Check sheet for the modelled part. Datum: model origin and axes. Units: mm. A direction names the side the tool comes from. Coordinates: 2 decimals unless noted, no trailing zeros. Order: outer loops, then holes, each group sorted by start corner. A loop starts at its lowest first (then second) coordinate and runs counter-clockwise, first axis right, second up.
from build123d import *

# Parameters (mm, degrees)
SKETCH_1_W      = 11.5
SKETCH_1_H      = 30
SKETCH_1_W_2    = 3
SKETCH_1_W_3    = 18.5
SKETCH_1_W_4    = 200
EXTRUDE_3_DEPTH = 5
FILLET_2_R      = 2


with BuildPart() as part:
    # 草图1 → 凸台-拉伸3 (new body)
    # profile 1 of 4: a face of its own
    with BuildSketch(Plane(origin=(0, 0, 0), x_dir=(0, 0, -1), z_dir=(1, 0, 0))):
        Rectangle(SKETCH_1_W, SKETCH_1_H)
        with BuildLine():
            Line((-1.75, -10), (-1.75, 10))
            ThreePointArc((-1.75, 10), (0, 11.75), (1.75, 10))
            Line((1.75, 10), (1.75, -10))
            ThreePointArc((1.75, -10), (0, -11.75), (-1.75, -10))
        make_face(mode=Mode.SUBTRACT)
    # profile 2 of 4: a face of its own
    with BuildSketch(Plane(origin=(0, 0, 0), x_dir=(0, 0, -1), z_dir=(1, 0, 0))):
        with Locations((-7.25, 0)):
            Rectangle(SKETCH_1_W_2, SKETCH_1_H)
    # profile 3 of 4: a face of its own
    with BuildSketch(Plane(origin=(0, 0, 0), x_dir=(0, 0, -1), z_dir=(1, 0, 0))):
        with Locations((15, 0)):
            Rectangle(SKETCH_1_W_3, SKETCH_1_H)
        with BuildLine():
            ThreePointArc((20.25, -10), (18.5, -11.75), (16.75, -10))
            Line((16.75, -10), (16.75, 10))
            ThreePointArc((16.75, 10), (18.5, 11.75), (20.25, 10))
            Line((20.25, 10), (20.25, -10))
        make_face(mode=Mode.SUBTRACT)
    # profile 4 of 4: a face of its own
    with BuildSketch(Plane(origin=(0, 0, 0), x_dir=(0, 0, -1), z_dir=(1, 0, 0))):
        with Locations((124.25, 0)):
            Rectangle(SKETCH_1_W_4, SKETCH_1_H)
        with BuildLine():
            ThreePointArc((36, -10), (34.25, -11.75), (32.5, -10))
            Line((32.5, -10), (32.5, 10))
            ThreePointArc((32.5, 10), (34.25, 11.75), (36, 10))
            Line((36, 10), (36, -10))
        make_face(mode=Mode.SUBTRACT)
        with BuildLine():
            ThreePointArc((51, -10), (49.25, -11.75), (47.5, -10))
            Line((47.5, -10), (47.5, 10))
            ThreePointArc((47.5, 10), (49.25, 11.75), (51, 10))
            Line((51, 10), (51, -10))
        make_face(mode=Mode.SUBTRACT)
        with BuildLine():
            ThreePointArc((196, -10), (194.25, -11.75), (192.5, -10))
            Line((192.5, -10), (192.5, 10))
            ThreePointArc((192.5, 10), (194.25, 11.75), (196, 10))
            Line((196, 10), (196, -10))
        make_face(mode=Mode.SUBTRACT)
        with BuildLine():
            ThreePointArc((207.5, 10), (209.25, 11.75), (211, 10))
            Line((211, 10), (211, -10))
            ThreePointArc((211, -10), (209.25, -11.75), (207.5, -10))
            Line((207.5, -10), (207.5, 10))
        make_face(mode=Mode.SUBTRACT)
    extrude(amount=EXTRUDE_3_DEPTH)

    # 圆角2
    fillet_2_edges = [part.edges().sort_by_distance(p)[0] for p in [
        (0, 0, 8.75),
    ]]
    fillet(fillet_2_edges, radius=FILLET_2_R)


solid = part.part
(1) Tool access check on faces 1 (the flat face through (0, 0, -107)), 2 (the flat face through (2, 0, -196)). Record the directions out of +Z, -Z, +X, -X, +Y, -Y that give a thin tool (end or side, any length) a straight path to the whole face; none if there is none.
Filled in:
face 1: +Z, -Z, -X, +Y, -Y
face 2: +X, -X
(2) Release check for a two-part mould opening along Y. For faces 3 (the flat face through (2, 0, -32.5)), 4 (the flat face through (2, 0, -224.25)), 5 (the flat face through (2, -15, -106)) record: +Y half, -Y half, draft (parallel to the pull), parting line (faces both ways), or undercut.
Filled in:
face 3: undercut
face 4: draft
face 5: -Y half
(3) Cross-section at B-B (x = 3.65). Enter the section's corners in (y, z).
Filled in:
outline: (-15, -224.25) - (15, -224.25) - (15, 8.75) - (-15, 8.75) - close; hole (-10, -211) - (10, -211) arc R1.75 ccw to (10, -207.5) - (-10, -207.5) arc R1.75 ccw to start; hole (-10, -196) - (10, -196) arc R1.75 ccw to (10, -192.5) - (-10, -192.5) arc R1.75 ccw to start; hole (-10, -51) - (10, -51) arc R1.75 ccw to (10, -47.5) - (-10, -47.5) arc R1.75 ccw to start; hole (-10, -36) - (10, -36) arc R1.75 ccw to (10, -32.5) - (-10, -32.5) arc R1.75 ccw to start; hole (-10, -20.25) - (10, -20.25) arc R1.75 ccw to (10, -16.75) - (-10, -16.75) arc R1.75 ccw to start; hole (-10, -1.75) - (10, -1.75) arc R1.75 ccw to (10, 1.75) - (-10, 1.75) arc R1.75 ccw to start
(4) Cross-section at A-A (y = -4.25). Count the separate pieces of the cut face and the enclosed holes in it, and give its area (3 significant figures).
Filled in:
separate pieces: 7
enclosed holes: 0
area: 1,060 mm2
(5) Thickness scan on probe 1 along Y at (x, z) = (1.4, -210.5); probe 2 along Y at (x, z) = (0.9, -19.5). Record the ranges inside material, lowest first.
Filled in:
probe 1: y = -15 to -11.22, 11.22 to 15
probe 2: y = -15 to -11.44, 11.44 to 15
